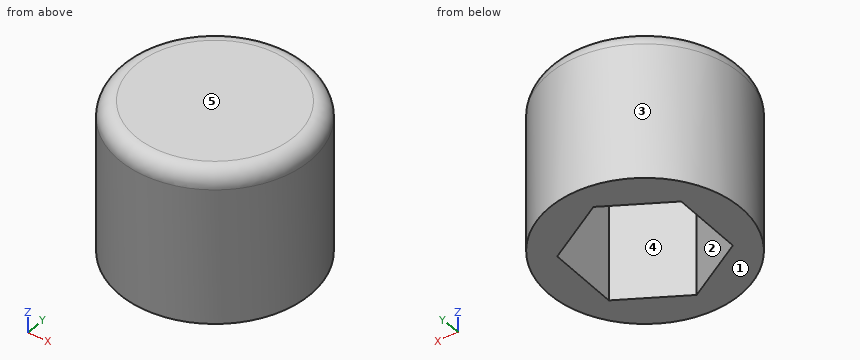
from build123d import *

# Parameters (mm, degrees)
F0_R     = 17.5
F1_DEPTH = 28
F2_DEPTH = 22
F3_R     = 3


with BuildPart() as f1:
    # F0 (on Top) → F1 (new body)
    with BuildSketch(Plane.XY):
        Circle(F0_R)
        Polygon((-11.25, 6.4951905284), (0, 12.9903810568), (11.25, 6.4951905284), (11.25, -6.4951905284), (0, -12.9903810568), (-11.25, -6.4951905284), align=None, mode=Mode.SUBTRACT)
        Polygon((11.25, 6.4951905284), (0, 12.9903810568), (-11.25, 6.4951905284), (-11.25, -6.4951905284), (0, -12.9903810568), (11.25, -6.4951905284), align=None)
    extrude(amount=F1_DEPTH)

    # F0 (on Top) → F2 (cut)
    with BuildSketch(Plane.XY):
        Polygon((11.25, 6.4951905284), (0, 12.9903810568), (-11.25, 6.4951905284), (-11.25, -6.4951905284), (0, -12.9903810568), (11.25, -6.4951905284), align=None)
    extrude(amount=F2_DEPTH, mode=Mode.SUBTRACT)

    # F3
    f3_edges = [f1.edges().sort_by_distance(p)[0] for p in [
        (-17.5, 0, 28),
    ]]
    fillet(f3_edges, radius=F3_R)


solid = f1.part
Geometry check sheet. Reference: the model listing, model coordinates, mm. Face numbers are marked on the shaded views. A direction names the side the tool comes from. Coordinates: 2 decimals unless noted, no trailing zeros. Order: outer loops, then holes, each group sorted by start corner. A loop starts at its lowest first (then second) coordinate and runs counter-clockwise, first axis right, second up. Notation, with made-up numbers: M 67.5,-34 L 122.5,-34 A27 ccw 122.5,-4 Z; hole C 61.5,59.25 d6. An arc over 180 degrees is marked long. Use CSV: the item, a comma, the result in double quotes.
Item 1: Cross-section at C-C on z = 24.5. Record the cut outline in (x, y).
Returned:
outline,"C 0,0 d35"
Item 2: Tool access check on the marked faces 1 and 2. Record the directions out of +Z, -Z, +X, -X, +Y, -Y that give a thin tool (end or side, any length) a straight path to the whole face; none if there is none.
Returned:
face 1,"-Z, +X, -X, +Y, -Y"
face 2,"-Z"
Item 3: Gauge pin test, flat ends, axial feed: pin 1 Ø5 at (y, z) = (3.5, 5) entering from +X; pin 2 Ø1.5 at (x, z) = (-3, 7.5) entering from +Y; pin 3 Ø1.5 at (x, z) = (-10, 20.5) entering from +Y. Record the tip position at first contact, or that the pin passes through.
Returned:
pin 1,"stops at x = 17.47"
pin 2,"stops at y = 17.35"
pin 3,"stops at y = 14.86"
Item 4: Thickness scan on line 1 along Y through (x, z) = (0, 6.75); line 2 along X through (y, z) = (0.5, 4); line 3 along Z through (x, y) = (9, -1.5). Record the ranges inside material, lowest first.
Returned:
line 1,"y = -17.5 to -12.99, 12.99 to 17.5"
line 2,"x = -17.49 to -11.25, 11.25 to 17.49"
line 3,"z = 22 to 28"
Item 5: Cross-section at B-B on y = 0. Record the cut outline in (x, z).
Returned:
outline,"M -17.5,0 L -11.25,0 L -11.25,22 L 11.25,22 L 11.25,0 L 17.5,0 L 17.5,25 A3 ccw 14.5,28 L -14.5,28 A3 ccw -17.5,25 Z"
Item 6: Mould release check, pull along X, two halves, no side actions. Record for the marked faces 3, 4 and 5: pulls with the +X half, pulls with the -X half, needs draft (parallel to the pull), parting line crosses it, or undercut.
Returned:
face 3,"parting line crosses it"
face 4,"undercut"
face 5,"needs draft"
Item 7: Cross-section at A-A on z = 21.5. Record the cut outline in (x, y).
Returned:
outline,"C 0,0 d35; hole M -11.25,-6.5 L 0,-12.99 L 11.25,-6.5 L 11.25,6.5 L 0,12.99 L -11.25,6.5 Z"
